Check sheet for the modelled part. Datum: model origin and axes. Units: mm. Face numbers are marked on the shaded views. A direction names the side the tool comes from. Round coordinates to 2 decimals unless told otherwise and drop trailing zeros. Write each loop counter-clockwise with the first axis right and the second up, starting at its lowest first coordinate (ties: lowest second). Pieces come first, ordered by that corner, then holes. Notation, with made-up numbers: (-28.5, -21.75) -> (-4.5, -21.75) arc R24 ccw to (-4.5, 0.25) -> close; hole circle Ø5 at (-6.75, 21.5). An arc over 180 degrees is marked (long way). Use one line per item in the form item = value. Start each with the question number.
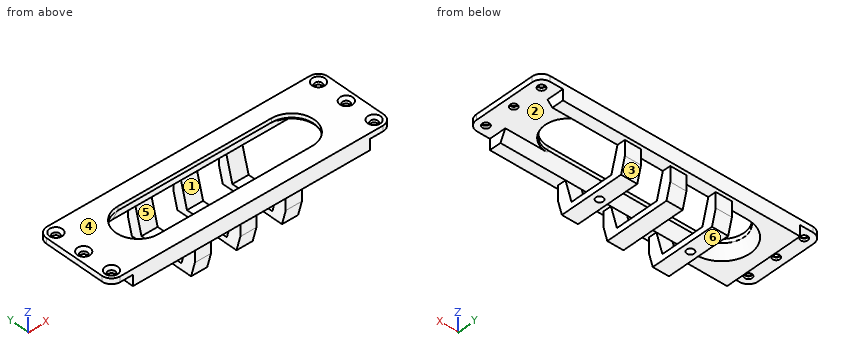
```python
from build123d import *

# Parameters (mm, degrees)
SKETCH1_W                = 118
SKETCH1_H                = 40
SKETCH1_W_2              = 11
BOSS_EXTRUDE1_DEPTH      = 3
BOSS_EXTRUDE2_START      = -5
SKETCH1_3_W              = 118
SKETCH1_3_H              = 40
BOSS_EXTRUDE2_DEPTH      = 5
FILLET1_R                = 5
CHAMFER1_SIZE            = 3
CHAMFER1_SIZE2           = 6
BOSS_EXTRUDE3_DEPTH      = 4
LPATTERN1_COUNT          = 2
LPATTERN1_PITCH          = 22.5
LPATTERN1_COL_COUNT      = 2
LPATTERN1_COL_PITCH      = 22.5
M3_CLEARANCE_HOLE1_D     = 3.6
M3_CLEARANCE_HOLE1_DEPTH = 9
M3_CLEARANCE_HOLE1_TIP   = 1.081549114
SKETCH9_W                = 53
SKETCH9_H                = 2
CUT_EXTRUDE1_DEPTH       = 75.34044996
CUT_EXTRUDE2_DEPTH       = 77.362965502
SKETCH12_W               = 5
SKETCH12_H               = 39.4
CUT_EXTRUDE3_DEPTH       = 0.3
SKETCH13_W               = 5
SKETCH13_H               = 39.4
CUT_EXTRUDE4_DEPTH       = 0.3
CUT_EXTRUDE5_START       = -0.3
CUT_EXTRUDE5_DEPTH       = 0.3
CUT_EXTRUDE6_DEPTH       = 30


# Read off the part's stored shape, not the designer's step: CSK for M3 Flat Head Machine Screw1
with BuildPart() as part:
    # Sketch1 → Boss-Extrude1 (new body)
    # profile 1 of 3: a face of its own
    with BuildSketch(Plane.XY):
        Rectangle(SKETCH1_W, SKETCH1_H)
        with BuildLine():
            ThreePointArc((-38, -11), (-49, 0), (-38, 11))
            Line((-38, 11), (38, 11))
            ThreePointArc((38, 11), (49, 0), (38, -11))
            Line((38, -11), (-38, -11))
        make_face(mode=Mode.SUBTRACT)
    # profile 2 of 3: a face of its own
    with BuildSketch(Plane.XY):
        with Locations((-64.5, 0)):
            Rectangle(SKETCH1_W_2, SKETCH1_H)
    # profile 3 of 3: a face of its own
    with BuildSketch(Plane.XY):
        with Locations((64.5, 0)):
            Rectangle(SKETCH1_W_2, SKETCH1_H)
    extrude(amount=BOSS_EXTRUDE1_DEPTH)

    # Sketch1<3> → Boss-Extrude2 (add)
    with BuildSketch(Plane.XY.offset(BOSS_EXTRUDE2_START)):
        Rectangle(SKETCH1_3_W, SKETCH1_3_H)
        with BuildLine():
            ThreePointArc((-38, -11), (-49, 0), (-38, 11))
            Line((-38, 11), (38, 11))
            ThreePointArc((38, 11), (49, 0), (38, -11))
            Line((38, -11), (-38, -11))
        make_face(mode=Mode.SUBTRACT)
    extrude(amount=BOSS_EXTRUDE2_DEPTH)

    # CSK for M3 Flat Head Machine Screw1 outl → CSK for M3 Flat Head Machine Screw1 (revolve, cut)
    with BuildSketch(Plane(origin=(65, 0, 0), x_dir=(1, 0, 0), z_dir=(0, -1, 0))):
        Polygon((0, 0), (1.8, 0), (1.8, 1.65), (3.15, 3), (0, 3), align=None)
    revolve(axis=Axis((65, 0, 0), (0, 0, 1)), mode=Mode.SUBTRACT)

    # CSK for M3 Flat Head Machine Screw1 2 ou → CSK for M3 Flat Head Machine Screw1 2 (revolve, cut)
    with BuildSketch(Plane(origin=(-65, 0, 0), x_dir=(1, 0, 0), z_dir=(0, -1, 0))):
        Polygon((0, 0), (1.8, 0), (1.8, 1.65), (3.15, 3), (0, 3), align=None)
    revolve(axis=Axis((-65, 0, 0), (0, 0, 1)), mode=Mode.SUBTRACT)

    # CSK for M3 Flat Head Machine Screw1 3 ou → CSK for M3 Flat Head Machine Screw1 3 (revolve, cut)
    with BuildSketch(Plane(origin=(-65, -15, 0), x_dir=(1, 0, 0), z_dir=(0, -1, 0))):
        Polygon((0, 0), (1.8, 0), (1.8, 1.65), (3.15, 3), (0, 3), align=None)
    revolve(axis=Axis((-65, -15, 0), (0, 0, 1)), mode=Mode.SUBTRACT)

    # CSK for M3 Flat Head Machine Screw1 4 ou → CSK for M3 Flat Head Machine Screw1 4 (revolve, cut)
    with BuildSketch(Plane(origin=(65, 15, 0), x_dir=(1, 0, 0), z_dir=(0, -1, 0))):
        Polygon((0, 0), (1.8, 0), (1.8, 1.65), (3.15, 3), (0, 3), align=None)
    revolve(axis=Axis((65, 15, 0), (0, 0, 1)), mode=Mode.SUBTRACT)

    # CSK for M3 Flat Head Machine Screw1 5 ou → CSK for M3 Flat Head Machine Screw1 5 (revolve, cut)
    with BuildSketch(Plane(origin=(65, -15, 0), x_dir=(1, 0, 0), z_dir=(0, -1, 0))):
        Polygon((0, 0), (1.8, 0), (1.8, 1.65), (3.15, 3), (0, 3), align=None)
    revolve(axis=Axis((65, -15, 0), (0, 0, 1)), mode=Mode.SUBTRACT)

    # CSK for M3 Flat Head Machine Screw1 6 ou → CSK for M3 Flat Head Machine Screw1 6 (revolve, cut)
    with BuildSketch(Plane(origin=(-65, 15, 0), x_dir=(1, 0, 0), z_dir=(0, -1, 0))):
        Polygon((0, 0), (1.8, 0), (1.8, 1.65), (3.15, 3), (0, 3), align=None)
    revolve(axis=Axis((-65, 15, 0), (0, 0, 1)), mode=Mode.SUBTRACT)

    # Fillet1
    fillet1_edges = [part.edges().sort_by_distance(p)[0] for p in [
        (-70, -20, 1.5),
        (-70, 20, 1.5),
        (70, 20, 1.5),
        (70, -20, 1.5),
    ]]
    fillet(fillet1_edges, radius=FILLET1_R)

    # Chamfer1
    chamfer1_edges = [part.edges().sort_by_distance(p)[0] for p in [
        (0, 11, -5),
        (49, 0, -5),
        (-49, 0, -5),
        (0, -11, -5),
    ]]
    chamfer1_side = [part.faces().sort_by_distance(p)[0] for p in [
        (0, 18.75404655, -5),
    ]]
    chamfer(chamfer1_edges, length=CHAMFER1_SIZE, length2=CHAMFER1_SIZE2, reference=chamfer1_side[0])

    # Sketch5 → Boss-Extrude3 (add, symmetric)
    with BuildSketch(Plane(origin=(0, 0, 0), x_dir=(0, 0, -1), z_dir=(1, 0, 0))):
        Polygon((5, -14), (5, -20), (20.050000007, -15.967364652), (20.050000007, 15.967364652), (5, 20), (5, 14), (17.050000007, 10.771212229), (17.050000007, -10.771212229), align=None)
    boss_extrude3 = extrude(amount=BOSS_EXTRUDE3_DEPTH, both=True)

    # LPattern1: Boss-Extrude3 ×2
    with Locations(*[(i * LPATTERN1_PITCH, 0, 0) for i in range(1, LPATTERN1_COUNT)]):
        add(boss_extrude3)

    # LPattern1 col: Boss-Extrude3 ×2
    with Locations(*[(-i * LPATTERN1_COL_PITCH, 0, 0) for i in range(1, LPATTERN1_COL_COUNT)]):
        add(boss_extrude3)

    # M3 Clearance Hole1
    with Locations(Plane(origin=(0, 0, -20.050000007), x_dir=(-1, 0, 0), z_dir=(0, 0, -1))):
        with Locations((-22.5, 0), (22.5, 0)):
            Hole(M3_CLEARANCE_HOLE1_D / 2, depth=M3_CLEARANCE_HOLE1_DEPTH)
            with Locations((0, 0, -(M3_CLEARANCE_HOLE1_DEPTH + M3_CLEARANCE_HOLE1_TIP / 2))):  # 118° drill point
                Cone(0, M3_CLEARANCE_HOLE1_D / 2, M3_CLEARANCE_HOLE1_TIP, mode=Mode.SUBTRACT)

    # Sketch9 → Cut-Extrude1 (cut, through all)
    with BuildSketch(Plane(origin=(0, 0, -5), x_dir=(-1, 0, 0), z_dir=(0, 0, -1))):
        with Locations((0, 19)):
            Rectangle(SKETCH9_W, SKETCH9_H)
        with Locations((0, -19)):
            Rectangle(SKETCH9_W, SKETCH9_H)
    extrude(amount=CUT_EXTRUDE1_DEPTH, mode=Mode.SUBTRACT)

    # Sketch10 → Cut-Extrude2 (cut, through all)
    with BuildSketch(Plane.XY.offset(3)):
        with BuildLine():
            Line((70, -15), (70, 15))
            ThreePointArc((70, 15), (68.535533906, 18.535533906), (65, 20))
            Line((65, 20), (-65, 20))
            ThreePointArc((-65, 20), (-68.535533906, 18.535533906), (-70, 15))
            Line((-70, 15), (-70, -15))
            ThreePointArc((-70, -15), (-68.535533906, -18.535533906), (-65, -20))
            Line((-65, -20), (65, -20))
            ThreePointArc((65, -20), (68.535533906, -18.535533906), (70, -15))
        make_face()
        with BuildLine():
            Line((69.7, -15), (69.7, 15))
            ThreePointArc((69.7, 15), (68.323401872, 18.323401872), (65, 19.7))
            Line((65, 19.7), (-65, 19.7))
            ThreePointArc((-65, 19.7), (-68.323401872, 18.323401872), (-69.7, 15))
            Line((-69.7, 15), (-69.7, -15))
            ThreePointArc((-69.7, -15), (-68.323401872, -18.323401872), (-65, -19.7))
            Line((-65, -19.7), (65, -19.7))
            ThreePointArc((65, -19.7), (68.323401872, -18.323401872), (69.7, -15))
        make_face(mode=Mode.SUBTRACT)
    extrude(amount=-CUT_EXTRUDE2_DEPTH, mode=Mode.SUBTRACT)

    # Sketch12 → Cut-Extrude3 (cut)
    with BuildSketch(Plane(origin=(59, 0, 0), x_dir=(0, 0, -1), z_dir=(1, 0, 0))):
        with Locations((2.5, 0)):
            Rectangle(SKETCH12_W, SKETCH12_H)
    extrude(amount=-CUT_EXTRUDE3_DEPTH, mode=Mode.SUBTRACT)

    # Sketch13 → Cut-Extrude4 (cut)
    with BuildSketch(Plane.ZY.offset(59)):
        with Locations((-2.5, 0)):
            Rectangle(SKETCH13_W, SKETCH13_H)
    extrude(amount=-CUT_EXTRUDE4_DEPTH, mode=Mode.SUBTRACT)

    # Sketch14 → Cut-Extrude5 (cut)
    with BuildSketch(Plane(origin=(0, 0, 0), x_dir=(-1, 0, 0), z_dir=(0, 0, -1)).offset(CUT_EXTRUDE5_START)):
        with BuildLine():
            Line((-65, -19.7), (-58.7, -19.7))
            Line((-58.7, -19.7), (-58.7, 19.7))
            Line((-58.7, 19.7), (-65, 19.7))
            ThreePointArc((-65, 19.7), (-68.323401872, 18.323401872), (-69.7, 15))
            Line((-69.7, 15), (-69.7, -15))
            ThreePointArc((-69.7, -15), (-68.323401872, -18.323401872), (-65, -19.7))
        make_face()
        with BuildLine():
            Line((58.7, -19.7), (65, -19.7))
            ThreePointArc((65, -19.7), (68.323401872, -18.323401872), (69.7, -15))
            Line((69.7, -15), (69.7, 15))
            ThreePointArc((69.7, 15), (68.323401872, 18.323401872), (65, 19.7))
            Line((65, 19.7), (58.7, 19.7))
            Line((58.7, 19.7), (58.7, -19.7))
        make_face()
    extrude(amount=CUT_EXTRUDE5_DEPTH, mode=Mode.SUBTRACT)

    # Sketch15 → Cut-Extrude6 (cut)
    with BuildSketch(Plane(origin=(58.7, 0, 0), x_dir=(0, 0, -1), z_dir=(1, 0, 0))):
        Polygon((-0.3, -11.35), (5, -14), (5, 14), (-0.3, 11.35), align=None)
    extrude(amount=-CUT_EXTRUDE6_DEPTH, mode=Mode.SUBTRACT)


solid = part.part
```
1. Sectioned sample at D-D (y = 7). Give the number of separate pieces and of enclosed holes in the cut face, and give its area (3 significant figures).
2. Sectioned sample at C-C (x = 51). Enter the section's corners in (y, z), and give its area (3 significant figures).
3. Mould release check, pull along Z, two halves, no side actions. Record for the marked faces 4, 5 and 6: +Z half, -Z half, draft (parallel to the pull), parting line (faces both ways), or undercut.
4. Scan lines: probe 1 along Y at (x, z) = (-65, 1.2); probe 2 along X at (y, z) = (15.5, -11.25); probe 3 along Y at (x, z) = (35, -0.75) (3 decimals). Record each from-to range of solid material in increasing order.
5. Tool access check on the marked faces 1, 2 and 3. Record the directions out of +Z, -Z, +X, -X, +Y, -Y that give a thin tool (end or side, any length) a straight path to the whole face; none if there is none.
6. Sectioned sample at B-B (z = -14.5). Enter the section's corners in (x, y).
7. Depth check by flat-ended pin: pin 1 (12 mm diameter, centred on x = -63, y = -9, fed in from -Z); pin 2 (6 mm diameter, centred on y = -6.5, z = -3, fed in from -X); pin 3 (5 mm diameter, centred on y = 7, z = -13.5, fed in from +X); pin 4 (6 mm diameter, centred on x = 65, y = -15, fed in from +Z). Enter the tip coordinate at first touch or a pass-through.
8. Sectioned sample at A-A (x = 22.5). Enter the section's corners in (y, z), and give its area (3 significant figures).
Returned:
q1.separate_pieces = 5
q1.enclosed_holes = 0
q1.area = 251 mm^2
q2.outline = (-19.7, -5) -> (-14, -5) -> (-11.35, 0.3) -> (11.35, 0.3) -> (14, -5) -> (19.7, -5) -> (19.7, 3) -> (-19.7, 3) -> close
q2.area = 181 mm^2
q3.face_4 = +Z half
q3.face_5 = undercut
q3.face_6 = -Z half
q4.probe_1 = -19.7 to -16.8, -13.2 to -1.8, 1.8 to 13.2, 16.8 to 19.7
q4.probe_2 = -26.5 to -18.5, -4 to 4, 18.5 to 26.5
q4.probe_3 = -19.7 to -11.875, 11.875 to 19.7
q5.face_1 = +X, -X
q5.face_2 = -Z, +X
q5.face_3 = -Z, +X, -X, +Y
q6.outline = (-26.5, -17.45) -> (-18.5, -17.45) -> (-18.5, -11.45) -> (-26.5, -11.45) -> close; (-26.5, 11.45) -> (-18.5, 11.45) -> (-18.5, 17.45) -> (-26.5, 17.45) -> close; (-4, -17.45) -> (4, -17.45) -> (4, -11.45) -> (-4, -11.45) -> close; (-4, 11.45) -> (4, 11.45) -> (4, 17.45) -> (-4, 17.45) -> close; (18.5, -17.45) -> (26.5, -17.45) -> (26.5, -11.45) -> (18.5, -11.45) -> close; (18.5, 11.45) -> (26.5, 11.45) -> (26.5, 17.45) -> (18.5, 17.45) -> close
q7.pin_1 = -5
q7.pin_2 = -58.7
q7.pin_3 = through
q7.pin_4 = 2.85
q8.outline = (-19.7, -5) -> (-18, -5) -> (-18, -12.46) -> (-15.97, -20.05) -> (-1.8, -20.05) -> (-1.8, -17.05) -> (-10.77, -17.05) -> (-14, -5) -> (-11, 1) -> (-11, 3) -> (-19.7, 3) -> close; (1.8, -20.05) -> (15.97, -20.05) -> (18, -12.46) -> (18, -5) -> (19.7, -5) -> (19.7, 3) -> (11, 3) -> (11, 1) -> (14, -5) -> (10.77, -17.05) -> (1.8, -17.05) -> close
q8.area = 338 mm^2
